from build123d import *

# Parameters (mm, degrees)
BOSS_EXTRUDE1_DEPTH = 66
CUT_EXTRUDE2_START  = -17
SKETCH3_R           = 22.5
SKETCH3_R_2         = 16.5
CUT_EXTRUDE2_DEPTH  = 13
CUT_EXTRUDE3_REACH  = 117.568
SKETCH3_2_R         = 16.5
CUT_EXTRUDE5_DEPTH  = 116.568161866


with BuildPart() as part:
    # Sketch1 → Boss-Extrude1 (new body)
    with BuildSketch(Plane.XY):
        with BuildLine():
            Line((0, 0), (30, 0))
            Line((30, 0), (30, 75))
            ThreePointArc((30, 75), (25.606601718, 85.606601718), (15, 90))
            Line((15, 90), (0, 90))
            Line((0, 90), (0, 0))
        make_face()
    extrude(amount=BOSS_EXTRUDE1_DEPTH)

    # Sketch3 → Cut-Extrude2 (cut)
    with BuildSketch(Plane(origin=(30, 0, 0), x_dir=(0, 0, -1), z_dir=(1, 0, 0)).offset(CUT_EXTRUDE2_START)):
        with Locations((-33, 35)):
            Circle(SKETCH3_R)
        with Locations((-33, 35)):
            Circle(SKETCH3_R_2, mode=Mode.SUBTRACT)
    extrude(amount=-CUT_EXTRUDE2_DEPTH, mode=Mode.SUBTRACT)

    # Sketch3<2> → Cut-Extrude3 (cut, up to next)
    with BuildSketch(Plane(origin=(30, 0, 0), x_dir=(0, 0, -1), z_dir=(1, 0, 0)), mode=Mode.PRIVATE) as cut_extrude3_sk1:
        with Locations((-33, 35)):
            Circle(SKETCH3_2_R)
    cut_extrude3_tool1 = extrude(cut_extrude3_sk1.sketch, amount=-CUT_EXTRUDE3_REACH, mode=Mode.PRIVATE) & part.part
    add(cut_extrude3_tool1.solids().sort_by_distance((30, 35, 33))[0], mode=Mode.SUBTRACT)

    # Cut-Loft1: read off the stored shape, not the designer's step
    # Cut-Loft1: loft between two sections, ruled curve by curve
    cut_loft1_from = [
        Edge.make_bspline([(8.104234717, 77.203503702, 66), (10.511242121, 90.995034268, 66), (24.302772687, 88.588026864, 66), (21.895765283, 74.796496298, 66), (19.488757879, 61.004965732, 66), (5.697227313, 63.411973136, 66), (8.104234717, 77.203503702, 66)], [0, 0, 0, 0, 0.5, 0.5, 0.5, 1, 1, 1, 1], 3, [1, 0.333333333, 0.333333333, 1, 0.333333333, 0.333333333, 1]),
    ]
    cut_loft1_to = [
        Edge.make_bspline([(9.125428786, 74.779584885, 0), (6.684598557, 86.528727313, 0), (18.433740984, 88.969557543, 0), (20.874571214, 77.220415115, 0), (23.315401443, 65.471272687, 0), (11.566259016, 63.030442457, 0), (9.125428786, 74.779584885, 0)], [0, 0, 0, 0, 0.5, 0.5, 0.5, 1, 1, 1, 1], 3, [1, 0.333333333, 0.333333333, 1, 0.333333333, 0.333333333, 1]),
    ]
    cut_loft1 = Solid(Shell([*[Face.make_surface_from_curves(cut_loft1_from[k], cut_loft1_to[k]) for k in range(1)], Face(Wire(cut_loft1_from)), Face(Wire(cut_loft1_to))]))
    add(cut_loft1, mode=Mode.SUBTRACT)

    # Sketch8 → Cut-Extrude5 (cut, through all)
    with BuildSketch(Plane.ZY):
        with BuildLine():
            ThreePointArc((33.000000237, 0), (16.323732633, 1.215545408), (0, 4.836485169))
            Line((0, 4.836485169), (0, 0))
            Line((0, 0), (33.000000237, 0))
        make_face()
        with BuildLine():
            ThreePointArc((66, 4.836485169), (49.676267601, 1.215545443), (33.000000237, 0))
            Line((33.000000237, 0), (66, 0))
            Line((66, 0), (66, 4.836485169))
        make_face()
    extrude(amount=-CUT_EXTRUDE5_DEPTH, mode=Mode.SUBTRACT)


solid = part.part
Build history of the part. All positions in model axes, mm. A direction names the side the tool comes from. Coordinates: 2 decimals unless noted, no trailing zeros. Write each loop counter-clockwise with the first axis right and the second up, starting at its lowest first coordinate (ties: lowest second). Pieces come first, ordered by that corner, then holes.
(1) Cut at A-A on y = 35. List the corners of the cut face in (x, z).
(2) Cut at B-B on x = 3. List the corners of the cut face in (y, z).
(3) Cut at C-C on z = 28. State how many separate pieces and enclosed holes the cut face has, and give its area (3 significant figures).
(4) 3-axis set-ups, long thin cutter, end or side, ignore diameter. For faces 1 (the flat face through (30, 54, 33)), 2 (the cylindrical face through (6.591, 13.035, 37.878)): which of +Z, -Z, +X, -X, +Y, -Y reach the whole face in a straight line?
(5) Drill centre lines: line 1 (Y direction, x = 1, z = 50); line 2 (Y direction, x = 23, z = 45); line 3 (X direction, y = 51, z = 21.5). Where is each one in solid material? Low to high.
(6) Pin check, flat tips, straight feed: pin 1 Ø13.5 at (y, z) = (33.5, 23.5) entering from -X; pin 2 Ø5 at (x, z) = (4, 30.5) entering from -Y; pin 3 Ø6 at (x, z) = (25.5, 53.5) entering from +Y; pin 4 Ø12 at (x, z) = (20, 8.5) entering from -Y. Stop position of each tip, or through.
(7) Mould opens along Y. For faces 3 (the flat face through (0, 56, 47)), 4 (the cylindrical face through (25.72, 85.49, 32.54)), 5 (the flat face through (13, 47, 45)) say: pulls with the +Y half, pulls with the -Y half, needs draft (parallel to the pull), parting line crosses it, or undercut.
(8) Cut at D-D on y = 46.5. List the corners of the cut face in (x, z).
Working result:
1. outline: (0, 0) - (30, 0) - (30, 16.5) - (13, 16.5) - (13, 10.5) - (0, 10.5) - close; (0, 55.5) - (13, 55.5) - (13, 49.5) - (30, 49.5) - (30, 66) - (0, 66) - close
2. outline: (4.84, 0) - (90, 0) - (90, 66) - (4.84, 66) arc R115 ccw to start; hole circle Ø45 at (35, 33)
3. separate pieces: 2
3. enclosed holes: 1
3. area: 1,420 mm2
4. face 1: +Z, -Z, +X, +Y, -Y
4. face 2: -X
5. line 1: y = 1.26 to 20.26, 49.74 to 90
5. line 2: y = 0.63 to 23.68, 46.32 to 87.69
5. line 3: x = 13 to 30
6. pin 1: passes through
6. pin 2: stops at y = 0
6. pin 3: stops at y = 87.99
6. pin 4: stops at y = 1.5
7. face 3: needs draft
7. face 4: pulls with the +Y half
7. face 5: undercut
8. outline: (0, 0) - (30, 0) - (30, 21.17) - (13, 21.17) - (13, 13.66) - (0, 13.66) - close; (0, 52.34) - (13, 52.34) - (13, 44.83) - (30, 44.83) - (30, 66) - (0, 66) - close
